from build123d import *

# Parameters (mm, degrees)
SKETCH1_R           = 3.175
BOSS_EXTRUDE1_DEPTH = 60.96
SKETCH2_R           = 1.5875
BOSS_EXTRUDE2_DEPTH = 12.7
CUT_EXTRUDE1_DEPTH  = 74.796726553


with BuildPart() as part:
    # Sketch1 → Boss-Extrude1 (new body)
    with BuildSketch(Plane(origin=(0, 0, 0), x_dir=(0, 0, -1), z_dir=(1, 0, 0))):
        with Locations(Location((0, 0, 0), (0, 0, 180))):
            Circle(SKETCH1_R)
    extrude(amount=BOSS_EXTRUDE1_DEPTH)

    # Sketch2 → Boss-Extrude2 (add)
    with BuildSketch(Plane(origin=(60.96, 0, 0), x_dir=(0, 0, -1), z_dir=(1, 0, 0))):
        Circle(SKETCH2_R)
    extrude(amount=BOSS_EXTRUDE2_DEPTH)

    # Sketch4 → Revolve1 (revolve)
    with BuildSketch(Plane.XY, mode=Mode.PRIVATE) as revolve1_sk:
        Polygon((60.96, -1.5875), (66.04, -1.5875), (66.04, -2.0447), (60.96, -3.175), align=None)
    revolve(revolve1_sk.sketch.rotate(Axis((60.96, 0, 0), (1, 0, 0)), 270), axis=Axis((60.96, 0, 0), (1, 0, 0)))

    # Sketch3 → Cut-Extrude1 (cut, through all)
    with BuildSketch(Plane.ZY):
        with BuildLine():
            Line((1.641398233, 2.7178), (-1.641398233, 2.7178))
            ThreePointArc((-1.641398233, 2.7178), (0, 3.175), (1.641398233, 2.7178))
        make_face()
    extrude(amount=-CUT_EXTRUDE1_DEPTH, mode=Mode.SUBTRACT)


solid = part.part
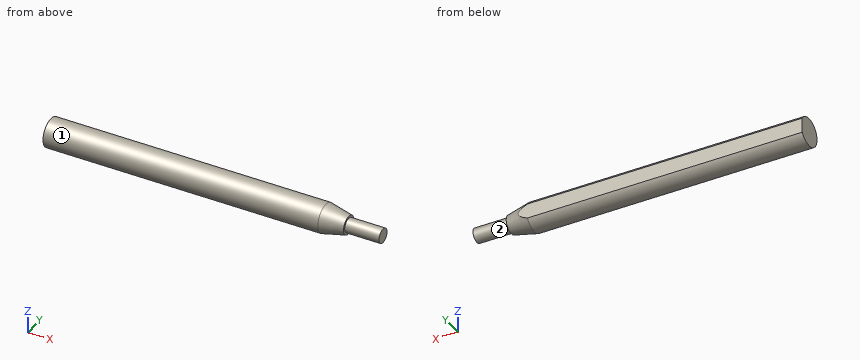
The listing builds one solid part. Answer for the finished solid, in the listing's coordinates (mm). Face numbers are marked on the shaded views. A direction names the side the tool comes from. Give positions to 0.01 mm unless a question says otherwise; leave off trailing zeros. Order: outer loops, then holes, each group sorted by start corner. A loop starts at its lowest first (then second) coordinate and runs counter-clockwise, first axis right, second up. Notation, with made-up numbers: (17.5, 44) - (25.5, 44) arc R19 cw to (25.5, 79) - close; hole circle Ø10 at (-39, 49.5). An arc over 180 degrees is marked (long way). One line per item, written item: value. Start each with the question number.
1) A tool of negligible diameter and unlimited length cuts with its end or side. For the marked faces 1 and 2, from which of +Z, -Z, +X, -X, +Y, -Y can it reach the whole face along a straight path? Write none if from no direction.
2) A cutting plane is placed at A-A on z = 0. Give the vertices of the cut face in (x, y) (1 decimal), then the cut area to 3 significant figures.
3) A cutting plane is placed at B-B on y = 0. Give the vertices of the cut face in (x, z) (1 decimal), then the cut area to 3 significant figures.
4) A cutting plane is placed at C-C on x = 59. Give the vertices of the cut face in (y, z) (3 decimals).
5) Find the intervals of material crossed by L1, parallel to X at y = 1.6, z = 0.5; L2, parallel to Y at x = 55.5, z = 1.25; L3, parallel to Z at x = 68, y = 0.2, in increasing order.
6) Given pin 1 Ø3 at (x, y) = (32, -2) entering from -Z, flat-ended and moving along its own axis, determine where the tip first touches the part or whether it passes through.
Answer sheet:
1. face 1: +X, -X
1. face 2: +X
2. outline: (0, -3.2) - (61, -3.2) - (66, -2) - (66, -1.6) - (73.7, -1.6) - (73.7, 1.6) - (66, 1.6) - (66, 2) - (63, 2.7) - (0, 2.7) - close
2. area: 409 mm2
3. outline: (0, -3.2) - (61, -3.2) - (66, -2) - (66, -1.6) - (73.7, -1.6) - (73.7, 1.6) - (66, 1.6) - (66, 2) - (61, 3.2) - (0, 3.2) - close
3. area: 438 mm2
4. outline: (2.718, -1.641) - (2.718, 1.641) arc R3.175 ccw (long way) to start
5. L1: x = 0 to 66.04
5. L2: y = -2.92 to 2.72
5. L3: z = -1.57 to 1.57
6. pin 1: stops at z = -3.14
